Verification items for this drawing (mm, ordinates from the low corner). A direction names the side the tool comes from. Give positions to 0.01 mm unless a question says otherwise; leave off trailing zeros. Write each loop counter-clockwise with the first axis right and the second up, starting at its lowest first coordinate (ties: lowest second). Pieces come first, ordered by that corner, then holes. Notation, with made-up numbers: M -40,-12.5 L -16,-12.5 A20 ccw -16,13.5 Z; hole C 19,42.5 d8. An arc over 180 degrees is marked long. Write each question's results on one line, items separated by ' | '.
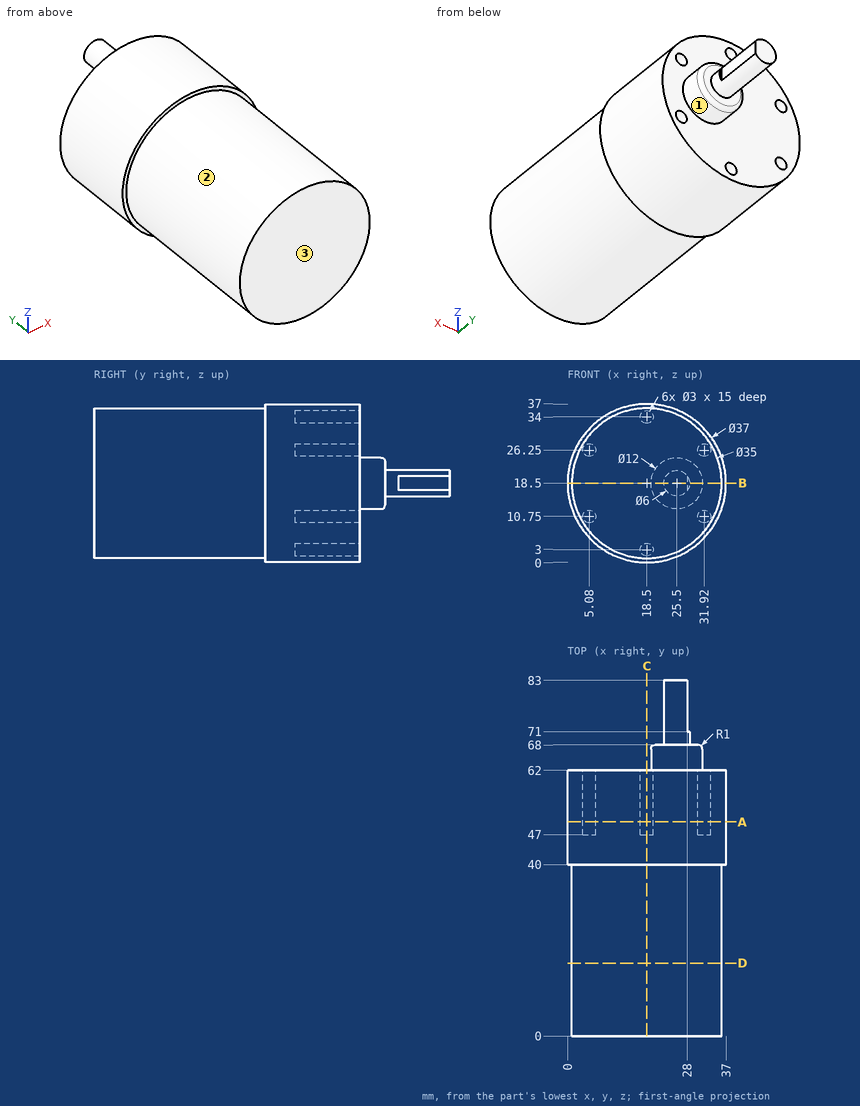
Q1. Section check B-B (z = 18.5). Enter the section's corners in (x, y), then the cut area to 3 significant figures.
Answer key:
outline: M 0,40 L 1,40 L 1,0 L 36,0 L 36,40 L 37,40 L 37,62 L 31.5,62 L 31.5,67 A1 ccw 30.5,68 L 28.5,68 L 28.5,71 L 28,71 L 28,83 L 22.5,83 L 22.5,68 L 20.5,68 A1 ccw 19.5,67 L 19.5,62 L 0,62 Z | area: 2,370 mm2
Q2. Access from +Z, -Z, +X, -X, +Y, -Y to the whole of each face (thin tool, end or side, straight path). Record for the marked faces 1, 2 and 3.
Answer key:
face 1: +Y | face 2: -Y | face 3: +Z, -Z, +X, -X, -Y
Q3. Depth check by flat-ended pin: P1, Ø1, axis at y = 35, z = 10, coming from the +X side; P2, Ø12, axis at x = 17, z = 25.5, coming from the +Y side; P3, Ø4, axis at x = 18.5, z = 3, coming from the +Y side. Enter the tip coordinate at first touch or a pass-through.
Answer key:
P1: stops at x = 34.06 | P2: stops at y = 68 | P3: stops at y = 62
Q4. Section check C-C (x = 18.5). Enter the section's corners in (y, z), then the cut area to 3 significant figures.
Answer key:
outline: M 0,1 L 40,1 L 40,0 L 62,0 L 62,1.5 L 47,1.5 L 47,4.5 L 62,4.5 L 62,32.5 L 47,32.5 L 47,35.5 L 62,35.5 L 62,37 L 40,37 L 40,36 L 0,36 Z | area: 2,120 mm2
Q5. Section check A-A (y = 50). Enter the section's corners in (x, z).
Answer key:
outline: C 18.5,18.5 d37; hole C 5.08,10.75 d3; hole C 5.08,26.25 d3; hole C 18.5,3 d3; hole C 18.5,34 d3; hole C 31.92,10.75 d3; hole C 31.92,26.25 d3
Q6. Section check D-D (y = 17). Enter the section's corners in (x, z), then the cut area to 3 significant figures.
Answer key:
outline: C 18.5,18.5 d35 | area: 962 mm2
Q7. Material ranges on probe 1 along X at (y, z) = (55, 10); probe 2 along Y at (x, z) = (3.5, 29); probe 3 along Y at (x, z) = (9.5, 5), recorded low to high. Write a range as [from, to].
Answer key:
probe 1: x = [2.07, 3.78], [6.38, 30.62], [33.22, 34.93] | probe 2: y = [40, 62] | probe 3: y = [0, 62]
